```python
from build123d import *

# Parameters (mm, degrees)
CUT_EXTRUDE1_DEPTH = 5.08


with BuildPart() as part:
    # Sketch1 → Revolve1 (revolve)
    with BuildSketch(Plane.XY):
        Polygon((0, -44.45), (25.4, -44.45), (25.4, -25.4), (30.1625, -25.4), (30.1625, 0), (33.3375, 0), (33.3375, -39.6875), (30.1625, -39.6875), (30.1625, -52.3875), (0, -52.3875), align=None)
    revolve(axis=Axis((0, -44.45, 0), (0, -1, 0)))

    # Sketch2 → Cut-Extrude1 (cut)
    with BuildSketch(Plane(origin=(0, -44.45, 0), x_dir=(1, 0, 0), z_dir=(0, 1, 0))):
        with BuildLine():
            Line((12.7, -15.875), (-12.7, -15.875))
            ThreePointArc((-12.7, -15.875), (-14.94506403, -14.94506403), (-15.875, -12.7))
            Line((-15.875, -12.7), (-15.875, 12.7))
            ThreePointArc((-15.875, 12.7), (-14.94506403, 14.94506403), (-12.7, 15.875))
            Line((-12.7, 15.875), (12.7, 15.875))
            ThreePointArc((12.7, 15.875), (14.94506403, 14.94506403), (15.875, 12.7))
            Line((15.875, 12.7), (15.875, -12.7))
            ThreePointArc((15.875, -12.7), (14.94506403, -14.94506403), (12.7, -15.875))
        make_face()
    extrude(amount=-CUT_EXTRUDE1_DEPTH, mode=Mode.SUBTRACT)


solid = part.part
```
Geometry: final body of the model. Coordinates: model frame, mm. A direction names the side the tool comes from. Round coordinates to 2 decimals unless told otherwise and drop trailing zeros. Order: outer loops, then holes, each group sorted by start corner. A loop starts at its lowest first (then second) coordinate and runs counter-clockwise, first axis right, second up. Notation, with made-up numbers: (-32, 57) -> (4, 57) arc R26 cw to (4, 92) -> close; hole circle Ø9 at (8, 39). An arc over 180 degrees is marked (long way). Write each question's results on one line, items separated by ' | '.
Q1. Pin query (flat end, axial travel): pin 1 Ø4 at (y, z) = (-42, -18.5) entering from +X; pin 2 Ø4 at (y, z) = (-47.5, 2.5) entering from +X; pin 3 Ø5 at (x, y) = (-16.5, -44) entering from +Z. Return the tip coordinate at first contact, or that it passes through.
Response values:
pin 1: x = 25.25 | pin 2: x = 30.16 | pin 3: z = 26.72
Q2. Pull-direction query (X, two-part tool) for faces 4 (the face through (31.8, -20.12, 10.01)), 5 (the face through (14.97, -46.95, 14.92)), 6 (the face through (-7.6, -39.688, -29.5)); classes: released by +X, released by -X, zero draft, split by the parting line, or undercut.
Response values:
face 4: split by the parting line | face 5: undercut | face 6: zero draft
Q3. Ray query, line 1 along Z through (x, y) = (0, -13.5); line 2 along Z through (x, y) = (0, -34.25); line 3 along Y through (x, z) = (-6, 16.5). Return the intervals inside material, ascending.
Response values:
line 1: -33.34 to -30.16, 30.16 to 33.34 | line 2: -33.34 to -25.4, 25.4 to 33.34 | line 3: -52.39 to -44.45
Q4. Section query D-D (z = 19.5). Output: boundary loops of the cut face in (x, y).
Response values:
outline: (-27.04, -39.69) -> (-23.01, -39.69) -> (-23.01, -52.39) -> (23.01, -52.39) -> (23.01, -39.69) -> (27.04, -39.69) -> (27.04, 0) -> (23.01, 0) -> (23.01, -25.4) -> (16.28, -25.4) -> (16.28, -44.45) -> (-16.28, -44.45) -> (-16.28, -25.4) -> (-23.01, -25.4) -> (-23.01, 0) -> (-27.04, 0) -> close
Q5. Section query C-C (y = -20). Output: boundary loops of the cut face in (x, z) (1 decimal).
Response values:
outline: circle Ø66.7 at (0, 0); hole circle Ø60.3 at (0, 0)
Q6. Access query for faces 1 (the face through (7.6, 0, -29.5)), 2 (the face through (15.875, -47, 0)), 3 (the face through (-30.133, -46.126, 1.326)). Directions: +Z, -Z, +X, -X, +Y, -Y. A direction counts if a zero-diameter tool reaches every point of the face in a straight line with its end or side. Return the directions, or none.
Response values:
face 1: +Z, -Z, +X, -X, +Y | face 2: +Y | face 3: -Y
